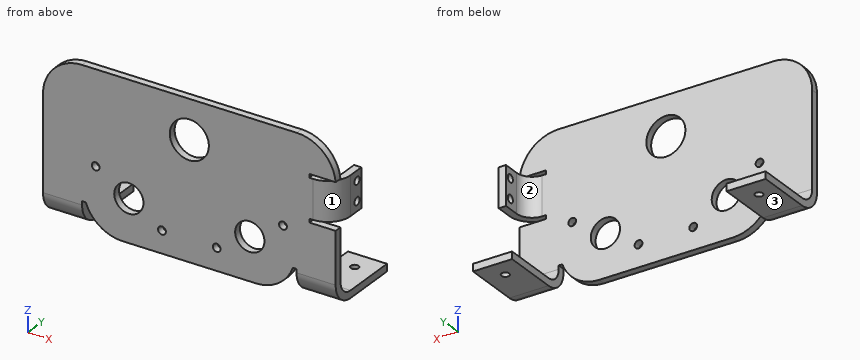
from build123d import *

# Parameters (mm, degrees)
SKETCH1_W                     = 190.5
SKETCH1_H                     = 101.6
BOSS_EXTRUDE1_DEPTH           = 1.5875
CONVERT_SOLID1_START          = -95.25
CONVERT_SOLID1_OUTLINE_W      = 3.175
CONVERT_SOLID1_OUTLINE_H      = 101.6
CONVERT_SOLID1_DEPTH          = 190.5
SKETCH35_W                    = 139.601875342
SKETCH35_H                    = 6.35
CUT_EXTRUDE7_DEPTH            = 0.254
EDGE_FLANGE1_STRIP_W          = 39.05
EDGE_FLANGE1_STRIP_H          = 4.7625
EDGE_FLANGE1_STRIP_CUT_DEPTH  = 25.449062329
EDGE_FLANGE1_RELIEF_W         = 41.43125
EDGE_FLANGE1_RELIEF_H         = 2.38125
EDGE_FLANGE1_RELIEF_CUT_DEPTH = 4.7625
EDGE_FLANGE1_DEPTH            = 25.449062329
EDGE_FLANGE2_STRIP_W          = 39.05
EDGE_FLANGE2_STRIP_H          = 4.7625
EDGE_FLANGE2_STRIP_CUT_DEPTH  = 25.449062329
EDGE_FLANGE2_RELIEF_W         = 41.43125
EDGE_FLANGE2_RELIEF_H         = 2.38125
EDGE_FLANGE2_RELIEF_CUT_DEPTH = 4.7625
EDGE_FLANGE2_DEPTH            = 25.449062329
SKETCH50_R                    = 12.713493351
CUT_EXTRUDE9_DEPTH            = 5.08
FILLET1_R                     = 25.4
CUT_EXTRUDE11_START           = -4.7625
CUT_EXTRUDE11_OUTLINE_W       = 6.35
CUT_EXTRUDE11_OUTLINE_H       = 0.00254
CUT_EXTRUDE11_OUTLINE_H_2     = 0.000254
CUT_EXTRUDE11_DEPTH           = 4.7625
EDGE_FLANGE3_STRIP_W          = 39.05
EDGE_FLANGE3_STRIP_H          = 4.7625
EDGE_FLANGE3_STRIP_CUT_DEPTH  = 25.4
EDGE_FLANGE3_RELIEF_W         = 41.43125
EDGE_FLANGE3_RELIEF_H         = 2.38125
EDGE_FLANGE3_RELIEF_CUT_DEPTH = 4.7625
EDGE_FLANGE3_DEPTH            = 25.4
SKETCH55_R                    = 2.54
CUT_EXTRUDE12_DEPTH           = 4.7625
FILLET2_R                     = 25.4
SKETCH56_R                    = 2.54
CUT_EXTRUDE13_DEPTH           = 4.7625
SKETCH57_R                    = 9.525
SKETCH57_R_2                  = 2.54
CUT_EXTRUDE14_DEPTH           = 4.7625


# Read off the part's stored shape, not the designer's step: Convert-Solid1, Cut-Extrude11
# Sheet-metal steps are written as plain solids
with BuildPart() as part:
    # Sketch1 → Boss-Extrude1 (new body)
    with BuildSketch(Plane(origin=(0, 0, 0), x_dir=(1, 0, 0), z_dir=(0, 1, 0))):
        Rectangle(SKETCH1_W, SKETCH1_H)
    extrude(amount=BOSS_EXTRUDE1_DEPTH)

    # Convert-Solid1 outline → Convert-Solid1 (add)
    with BuildSketch(Plane.YZ.offset(CONVERT_SOLID1_START)):
        with Locations((-1.5875, 0)):
            Rectangle(CONVERT_SOLID1_OUTLINE_W, CONVERT_SOLID1_OUTLINE_H)
    extrude(amount=CONVERT_SOLID1_DEPTH)

    # Sketch35 → Cut-Extrude7 (cut)
    with BuildSketch(Plane(origin=(0, 0, -50.8), x_dir=(-1, 0, 0), z_dir=(0, 0, -1))):
        Rectangle(SKETCH35_W, SKETCH35_H)
    extrude(amount=-CUT_EXTRUDE7_DEPTH, mode=Mode.SUBTRACT)

    # Edge-Flange1 strip (across the edge) → Edge-Flange1 strip cut (cut)
    with BuildSketch(Plane(origin=(95.25, 1.5875, -50.8), x_dir=(0, 0, 1), z_dir=(-1, 0, 0))):
        with Locations((-4.7625, -2.38125)):
            Rectangle(EDGE_FLANGE1_STRIP_W, EDGE_FLANGE1_STRIP_H)
    extrude(amount=EDGE_FLANGE1_STRIP_CUT_DEPTH, mode=Mode.SUBTRACT)

    # Edge-Flange1 relief (on the sheet) → Edge-Flange1 relief cut (cut)
    with BuildSketch(Plane(origin=(95.25, 1.5875, -36.0375), x_dir=(0, 0, 1), z_dir=(0, 1, 0))):
        with Locations((-18.334375, -26.639687329)):
            Rectangle(EDGE_FLANGE1_RELIEF_W, EDGE_FLANGE1_RELIEF_H)
    extrude(amount=-EDGE_FLANGE1_RELIEF_CUT_DEPTH, mode=Mode.SUBTRACT)

    # Edge-Flange1 section (across the edge) → Edge-Flange1 (add)
    with BuildSketch(Plane(origin=(95.25, 1.5875, -50.8), x_dir=(0, 0, 1), z_dir=(-1, 0, 0))):
        with BuildLine():
            Line((0, 10), (0, 46.0375))
            Line((0, 46.0375), (4.7625, 46.0375))
            Line((4.7625, 46.0375), (4.7625, 10))
            ThreePointArc((4.7625, 10), (7.691432188, 2.928932188), (14.7625, 0))
            Line((14.7625, 0), (14.7625, -4.7625))
            ThreePointArc((14.7625, -4.7625), (4.323836143, -0.438663857), (0, 10))
        make_face()
    extrude(amount=EDGE_FLANGE1_DEPTH)

    # Edge-Flange2 strip (across the edge) → Edge-Flange2 strip cut (cut)
    with BuildSketch(Plane(origin=(-69.800937671, 1.5875, -50.8), x_dir=(0, 0, 1), z_dir=(-1, 0, 0))):
        with Locations((-4.7625, -2.38125)):
            Rectangle(EDGE_FLANGE2_STRIP_W, EDGE_FLANGE2_STRIP_H)
    extrude(amount=EDGE_FLANGE2_STRIP_CUT_DEPTH, mode=Mode.SUBTRACT)

    # Edge-Flange2 relief (on the sheet) → Edge-Flange2 relief cut (cut)
    with BuildSketch(Plane(origin=(-69.800937671, 1.5875, -36.0375), x_dir=(0, 0, 1), z_dir=(0, 1, 0))):
        with Locations((-18.334375, 1.190625)):
            Rectangle(EDGE_FLANGE2_RELIEF_W, EDGE_FLANGE2_RELIEF_H)
    extrude(amount=-EDGE_FLANGE2_RELIEF_CUT_DEPTH, mode=Mode.SUBTRACT)

    # Edge-Flange2 section (across the edge) → Edge-Flange2 (add)
    with BuildSketch(Plane(origin=(-69.800937671, 1.5875, -50.8), x_dir=(0, 0, 1), z_dir=(-1, 0, 0))):
        with BuildLine():
            Line((0, 10), (0, 46.0375))
            Line((0, 46.0375), (4.7625, 46.0375))
            Line((4.7625, 46.0375), (4.7625, 10))
            ThreePointArc((4.7625, 10), (7.691432188, 2.928932188), (14.7625, 0))
            Line((14.7625, 0), (14.7625, -4.7625))
            ThreePointArc((14.7625, -4.7625), (4.323836143, -0.438663857), (0, 10))
        make_face()
    extrude(amount=EDGE_FLANGE2_DEPTH)

    # Sketch50 → Cut-Extrude9 (cut)
    with BuildSketch(Plane(origin=(0, -3.175, 0), x_dir=(-1, 0, 0), z_dir=(0, -1, 0))):
        with Locations(Location((0, -25.4, 0), (0, 0, 90))):
            Circle(SKETCH50_R)
    extrude(amount=-CUT_EXTRUDE9_DEPTH, mode=Mode.SUBTRACT)

    # Fillet1
    # the kernel refuses this fillet: 25.4 mm, written as the material it takes off along each edge
    with BuildSketch(Plane(origin=(-67.419687671, 61.417239936, -50.546), x_dir=(1, 0, 0), z_dir=(0, -1, 0))) as fillet1_piece_1:
        with BuildLine():
            CenterArc((23.931895975, 25.4), FILLET1_R, 199.575530564, 70.424469436)
            Line((0, 16.88975), (-0.478637919, 16.719545))
            ThreePointArc((-0.478637919, 16.719545), (-0.508, 8.444875), (-0.508, 0))
            Line((-0.508, 0), (0, -0.508))
            Line((0, -0.508), (23.931895975, -0.508))
            Line((23.931895975, -0.508), (23.931895975, 0))
        make_face()
    extrude(amount=124.421979873, mode=Mode.SUBTRACT)
    with BuildSketch(Plane(origin=(67.419687671, 61.417239936, -50.546), x_dir=(0, 0, 1), z_dir=(0, -1, 0))) as fillet1_piece_2:
        with BuildLine():
            CenterArc((25.4, 23.931895975), FILLET1_R, 180, 70.424469436)
            Line((0, 23.931895975), (-0.508, 23.931895975))
            Line((-0.508, 23.931895975), (-0.508, 0))
            Line((-0.508, 0), (0, -0.508))
            ThreePointArc((0, -0.508), (8.444875, -0.508), (16.719545, -0.478637919))
            Line((16.719545, -0.478637919), (16.88975, 0))
        make_face()
    extrude(amount=124.421979873, mode=Mode.SUBTRACT)

    # Cut-Extrude11 outline → Cut-Extrude11 (cut)
    with BuildSketch(Plane.XZ.offset(3.175).offset(CUT_EXTRUDE11_START)):
        with Locations((92.075, -0.001524)):
            Rectangle(CUT_EXTRUDE11_OUTLINE_W, CUT_EXTRUDE11_OUTLINE_H)
        with Locations((92.075, 25.399873)):
            Rectangle(CUT_EXTRUDE11_OUTLINE_W, CUT_EXTRUDE11_OUTLINE_H_2)
    extrude(amount=CUT_EXTRUDE11_DEPTH, mode=Mode.SUBTRACT)

    # Edge-Flange3 strip (across the edge) → Edge-Flange3 strip cut (cut)
    with BuildSketch(Plane(origin=(95.25, 1.5875, 25.399746), x_dir=(-1, 0, 0), z_dir=(0, 0, -1))):
        with Locations((-4.7625, -2.38125)):
            Rectangle(EDGE_FLANGE3_STRIP_W, EDGE_FLANGE3_STRIP_H)
    extrude(amount=EDGE_FLANGE3_STRIP_CUT_DEPTH, mode=Mode.SUBTRACT)

    # Edge-Flange3 relief (on the sheet) → Edge-Flange3 relief cut (cut)
    with BuildSketch(Plane(origin=(80.4875, 1.5875, 25.399746), x_dir=(-1, 0, 0), z_dir=(0, 1, 0))):
        with Locations((-18.334375, 1.190625)):
            Rectangle(EDGE_FLANGE3_RELIEF_W, EDGE_FLANGE3_RELIEF_H)
        with Locations((-18.334375, -26.590625)):
            Rectangle(EDGE_FLANGE3_RELIEF_W, EDGE_FLANGE3_RELIEF_H)
    extrude(amount=-EDGE_FLANGE3_RELIEF_CUT_DEPTH, mode=Mode.SUBTRACT)

    # Edge-Flange3 section (across the edge) → Edge-Flange3 (add)
    with BuildSketch(Plane(origin=(95.25, 1.5875, 25.399746), x_dir=(-1, 0, 0), z_dir=(0, 0, -1))):
        with BuildLine():
            Line((0, 10), (0, 20.6375))
            Line((0, 20.6375), (4.7625, 20.6375))
            Line((4.7625, 20.6375), (4.7625, 10))
            ThreePointArc((4.7625, 10), (7.691432188, 2.928932188), (14.7625, 0))
            Line((14.7625, 0), (14.7625, -4.7625))
            ThreePointArc((14.7625, -4.7625), (4.323836143, -0.438663857), (0, 10))
        make_face()
    extrude(amount=EDGE_FLANGE3_DEPTH)

    # Sketch55 → Cut-Extrude12 (cut)
    with BuildSketch(Plane(origin=(95.25, 0, 0), x_dir=(0, 0, -1), z_dir=(1, 0, 0))):
        with Locations(Location((-6.349746, 17.9375, 0), (0, 0, 90))):
            Circle(SKETCH55_R)
        with Locations(Location((-19.049746, 17.9375, 0), (0, 0, 90))):
            Circle(SKETCH55_R)
    extrude(amount=-CUT_EXTRUDE12_DEPTH, mode=Mode.SUBTRACT)

    # Fillet2
    # the kernel refuses this fillet: 25.4 mm, written as the material it takes off along each edge
    with BuildSketch(Plane(origin=(-95.25, 65.0875, 50.8), x_dir=(1, 0, 0), z_dir=(0, -1, 0))) as fillet2_piece_1:
        with BuildLine():
            CenterArc((FILLET2_R, -FILLET2_R), FILLET2_R, 90, 90)
            Line((0, -FILLET2_R), (-FILLET2_R * 0.02, -FILLET2_R))
            Line((-FILLET2_R * 0.02, -FILLET2_R), (-FILLET2_R * 0.02, FILLET2_R * 0.02))
            Line((-FILLET2_R * 0.02, FILLET2_R * 0.02), (FILLET2_R, FILLET2_R * 0.02))
            Line((FILLET2_R, FILLET2_R * 0.02), (FILLET2_R, 0))
        make_face()
    extrude(amount=131.7625, mode=Mode.SUBTRACT)
    with BuildSketch(Plane(origin=(95.25, -66.395391195, 50.8), x_dir=(-1, 0, 0), z_dir=(0, 1, 0))) as fillet2_piece_2:
        with BuildLine():
            CenterArc((25.288156478, -25.4), FILLET2_R, 90, 84.621196501)
            Line((0, -23.019004), (-0.50576313, -22.97138408))
            ThreePointArc((-0.50576313, -22.97138408), (-0.508, -11.509502), (-0.508, 0))
            Line((-0.508, 0), (0, 0.508))
            Line((0, 0.508), (25.288156478, 0.508))
            Line((25.288156478, 0.508), (25.288156478, 0))
        make_face()
    extrude(amount=131.203282389, mode=Mode.SUBTRACT)

    # Sketch56 → Cut-Extrude13 (cut)
    with BuildSketch(Plane(origin=(0, 0, -50.8), x_dir=(-1, 0, 0), z_dir=(0, 0, -1))):
        with Locations(Location((-82.55, 34.925, 0), (0, 0, 90))):
            Circle(SKETCH56_R)
        with Locations(Location((82.55, 34.925, 0), (0, 0, 90))):
            Circle(SKETCH56_R)
    extrude(amount=-CUT_EXTRUDE13_DEPTH, mode=Mode.SUBTRACT)

    # Sketch57 → Cut-Extrude14 (cut)
    with BuildSketch(Plane.XZ.offset(3.175)):
        with Locations(Location((39.37, -22.793111541, 0), (0, 0, 270))):
            Circle(SKETCH57_R)
        with Locations(Location((60.96, -9.412831275, 0), (0, 0, 270))):
            Circle(SKETCH57_R_2)
        with Locations(Location((17.801190198, -36.207523333, 0), (0, 0, 270))):
            Circle(SKETCH57_R_2)
        with Locations(Location((-17.801190198, -36.207523333, 0), (0, 0, 270))):
            Circle(SKETCH57_R_2)
        with Locations(Location((-39.37, -22.793111541, 0), (0, 0, 270))):
            Circle(SKETCH57_R)
        with Locations(Location((-60.96, -9.412831275, 0), (0, 0, 270))):
            Circle(SKETCH57_R_2)
    extrude(amount=-CUT_EXTRUDE14_DEPTH, mode=Mode.SUBTRACT)


solid = part.part
Read the model definition and answer for the solid it produces. Units are mm, in the model's axes. Face numbers are marked on the shaded views. A direction names the side the tool comes from. Coordinates: 2 decimals unless noted, no trailing zeros. Write each loop counter-clockwise with the first axis right and the second up, starting at its lowest first coordinate (ties: lowest second). Pieces come first, ordered by that corner, then holes. Notation, with made-up numbers: M -31,-37.75 L -8,-37.75 A31 cw -8,-8.75 Z; hole C -40,45.25 d4. An arc over 180 degrees is marked long. Use a Markdown table: item, result.
Q1. The part is cut by section B-B, the plane y = 30.5. Write down the section's boundary in (x, z).
Answer block:
| item | result |
|---|---|
| outline | M -95.25,-50.8 L -69.8,-50.8 L -69.8,-46.04 L -95.25,-46.04 Z; M 69.8,-50.8 L 95.25,-50.8 L 95.25,-46.04 L 69.8,-46.04 Z |
Q2. The part is cut by section A-A, the plane x = 39.37. Write down the section's boundary in (y, z) (1 decimal), then the cut area to 3 significant figures.
Answer block:
| item | result |
|---|---|
| outline | M -3.2,-50.5 L 1.6,-50.5 L 1.6,-32.3 L -3.2,-32.3 Z; M -3.2,-13.3 L 1.6,-13.3 L 1.6,50.8 L -3.2,50.8 Z |
| area | 392 mm2 |
Q3. Which of the six approach directions +Z, -Z, +X, -X, +Y, -Y give full straight-line access (tool end or side, diameter ignored) to the marked faces 1, 2 and 3?
Answer block:
| item | result |
|---|---|
| face 1 | +X, -Y |
| face 2 | +Z, -X, +Y |
| face 3 | -Z, +X, -X, +Y, -Y |
Q4. Each of these flat-tipped pins is pushed along its axis until it touches: pin 1 Ø1 at (x, z) = (13, -28) entering from +Y; pin 2 Ø2.5 at (x, z) = (92, 18.5) entering from +Y (3 decimals); pin 3 Ø4 at (x, y) = (86, -1.5) entering from +Z. Where does it stop, or does it pass through?
Answer block:
| item | result |
|---|---|
| pin 1 | stops at y = 1.59 |
| pin 2 | stops at y = 22.225 |
| pin 3 | stops at z = 46.57 |
Q5. The part is cut by section C-C, the plane x = 82.55. Write down the section's boundary in (y, z) (1 decimal).
Answer block:
| item | result |
|---|---|
| outline | M -3.2,-36 A14.8 ccw 11.6,-50.8 L 32.4,-50.8 L 32.4,-46 L 11.6,-46 A10 cw 1.6,-36 L 1.6,-2.4 L -3.2,-2.4 Z; M -3.2,27.8 L 1.6,27.8 L 1.6,47.5 L -3.2,47.5 Z; M -3,0 L 1.8,0 L 1.8,25.4 L -3,25.4 Z; M 37.5,-50.8 L 47.6,-50.8 L 47.6,-46 L 37.5,-46 Z |
Q6. Straight lines are drawn through the part: L1, parallel to Z at x = 39, y = 0; L2, parallel to Y at x = -37.5, z = 30 (1 decimal); L3, parallel to Y at x = 82, z = -48 (3 decimals). For each, find the intervals that lie inside material, in ascending order. Write a range as [from, to].
Answer block:
| item | result |
|---|---|
| L1 | z = [-50.55, -32.31], [-13.28, 50.8] |
| L2 | y = [-3.2, 1.6] |
| L3 | y = [2.937, 32.445], [37.405, 47.625] |
